Source: CAD feature listing. Evaluate the final solid. Frame: model axes, mm. A direction names the side the tool comes from. Coordinates: 2 decimals unless noted, no trailing zeros. Write each loop counter-clockwise with the first axis right and the second up, starting at its lowest first coordinate (ties: lowest second). Pieces come first, ordered by that corner, then holes. Notation, with made-up numbers: (-11, 76.25) -> (41, 76.25) arc R21 ccw to (41, 91.25) -> close; hole circle Ø4 at (53, -0.75). An arc over 180 degrees is marked (long way). One line per item, written item: value. Start each with the question number.
1. Mould query, pull axis X, two halves, no side actions, for faces 1 (the cylindrical face through (12.248, 5.151, -17.732)), 2 (the flat face through (0, 0, 2)), 3 (the flat face through (15, 0, -18)). Classes: released by +X, released by -X, zero draft, split by the parting line, or undercut.
2. Access query for faces 4 (the flat face through (5, 0, -7)), 5 (the cylindrical face through (-2.598, -3.237, 0.986)), 6 (the cylindrical face through (-4.4, 9.93, 1.01)), 7 (the flat face through (-2, 0, 0)), 8 (the flat face through (-8, 0, -18)). Directions: +Z, -Z, +X, -X, +Y, -Y. A direction counts if a zero-diameter tool reaches every point of the face in a straight line with its end or side. Return the directions, or none.
3. Section query C-C, the plane z = -4.5. Output: boundary loops of the cut face in (x, y).
4. Section query B-B, the plane y = -5.25. Output: boundary loops of the cut face in (x, z), and give its area (3 significant figures).
5. First-contact query: P1, Ø9, axis at y = 2, z = -10.5, coming from the +X side; P2, Ø1.9, axis at x = -2.26, y = 4.75, coming from the +Z side; P3, Ø8, axis at x = 12, z = -0.5, coming from the -Y side; P4, Ø1, axis at y = 1, z = 1.5, coming from the -X side. Flat tips, straight axial feed; report the tip coordinate or a pass-through.
6. Line query: line 1 (Y direction, x = 10, z = -17.75); line 2 (X direction, y = -5.25, z = -18.25); line 3 (Z direction, x = 0.75, y = 5.5). Output: solid intervals per line, ascending.
7. Section query A-A, the plane x = 10. Output: boundary loops of the cut face in (y, z), and give its area (3 significant figures).
Autodesk Fusion 360 part; units mm, degrees
sketch "Sketch1" plane through (0, 0, 0) normal (0, 0, 1) x (1, 0, 0)
  line L0 (5, 10.5) -> (-5, 10.5)
  line L1 (-5, 10.5) -> (-5, -10.5)
  line L2 (-5, -10.5) -> (5, -10.5)
  line L3 (5, -10.5) -> (5, 10.5)
  line L4 (5, 10.5) -> (-5, -10.5) construction
  line L5 (-5, 10.5) -> (5, -10.5) construction
  line L6 (5, -4.75) -> (-5, -4.75)
  line L7 (-5, -4.75) -> (-5, 4.75)
  line L8 (-5, 4.75) -> (5, 4.75)
  line L9 (5, 4.75) -> (5, -4.75)
  line L10 (5, -4.75) -> (-5, 4.75) construction
  line L11 (-5, -4.75) -> (5, 4.75) construction
  circle A0 centre (-2.2619, 4.75) radius 1.55
  circle A1 centre (-2.2619, -4.75) radius 1.55
  line L12 (5, 10.5) -> (2, 10.5)
  line L13 (2, 10.5) -> (2, -10.5)
  line L14 (2, -10.5) -> (5, -10.5)
  line L15 (5, -10.5) -> (5, 10.5)
  dimension "d1" = 10
  dimension "d2" = 21
  dimension "d3" = 10
  dimension "d4" = 9.5
  dimension "d5" = 3.1
  dimension "d6" = 3.1
  dimension "d7" = 3
extrude "Extrude1" add sketch "Sketch1" along normal blind 2 contours L0 L3 L8 L12 L13 L15 | L0 L1 L8 A0 L13 | L3 L6 L8 L9 L13 L15 | L1 L6 L7 L8 A0 A1 L13 | L2 L3 L6 L13 L14 L15 | L1 L2 L6 A1 L13
extrude "Extrude2" add sketch "Sketch1" against normal blind 19 contours L0 L3 L8 L12 L13 L15 | L3 L6 L8 L9 L13 L15 | L2 L3 L6 L13 L14 L15
sketch "Sketch2" plane through (5, 0, 0) normal (1, 0, 0) x (0, 1, 0)
  line L0 (10.5, -19) -> (10.5, 2)
  line L1 (10.5, 2) -> (-10.5, 2)
  line L2 (-10.5, 2) -> (-10.5, -19)
  line L3 (-10.5, -19) -> (10.5, -19)
  line L4 (-10.5, -19) -> (10.5, -19)
  line L5 (10.5, -19) -> (10.5, -16.5)
  line L6 (10.5, -16.5) -> (-10.5, -16.5)
  line L7 (-10.5, -16.5) -> (-10.5, -19)
  dimension "d12" = 2.5
extrude "Extrude3" add sketch "Sketch2" along normal blind 10 and the other way blind 13 contours L0 L2 L3 L4 L5 L6 L7
sketch "Sketch3" plane through (0, 0, -16.5) normal (0, 0, 1) x (-1, 0, 0)
  line L0 (-5, -10.5) -> (-5, 10.5)
  line L1 (-5, 10.5) -> (-15, 10.5)
  line L2 (-15, 10.5) -> (-15, -10.5)
  line L3 (-15, -10.5) -> (-5, -10.5)
  line L4 (-10, -10.5) -> (-10, 10.5)
  line L5 (-15, 0) -> (-5, 0)
  line L6 (-10, 0) -> (-10, -10.5)
  circle A0 centre (-10, -5.25) radius 2.25
  line L7 (-10, 0) -> (-10, 10.5)
  circle A1 centre (-10, 5.25) radius 2.25
  dimension "d17" = 4.5
  dimension "d18" = 4.5
fillet "Fillet1" radius 2 6 edges at (15, -10.5, -17.75) (15, 10.5, -17.75) (-8, -10.5, -17.75) (-5, -10.5, 1) (-5, 10.5, 1) (-8, 10.5, -17.75)
extrude "Extrude4" cut sketch "Sketch3" against normal blind 7 contours L4 L6 A0 | L4 L6 A0 | L4 L7 A1 | L4 L7 A1
Computed values:
1. face 1: undercut
1. face 2: zero draft
1. face 3: released by +X
2. face 4: +Z, +X, +Y, -Y
2. face 5: +Z
2. face 6: +Z, -X, +Y
2. face 7: -X, +Y, -Y
2. face 8: +Z, -Z, -X, +Y, -Y
3. outline: (2, -10.5) -> (5, -10.5) -> (5, 10.5) -> (2, 10.5) -> close
4. outline: (-8, -19) -> (7.75, -19) -> (7.75, -16.5) -> (5, -16.5) -> (5, 2) -> (-0.79, 2) -> (-0.79, 0) -> (2, 0) -> (2, -16.5) -> (-8, -16.5) -> close; (-5, 0) -> (-3.73, 0) -> (-3.73, 2) -> (-5, 2) -> close; (12.25, -19) -> (15, -19) -> (15, -16.5) -> (12.25, -16.5) -> close
4. area: 110 mm²
5. P1: stops at x = 5
5. P2: stops at z = -16.5
5. P3: passes through
5. P4: stops at x = -5
6. line 1: y = -10.5 to -7.5, -3 to 3, 7.5 to 10.5
6. line 2: x = -8 to 7.75, 12.25 to 15
6. line 3: z = -19 to -16.5, 0 to 2
7. outline: (-10.5, -19) -> (-7.5, -19) -> (-7.5, -16.5) -> (-10.5, -16.5) -> close; (-3, -19) -> (3, -19) -> (3, -16.5) -> (-3, -16.5) -> close; (7.5, -19) -> (10.5, -19) -> (10.5, -16.5) -> (7.5, -16.5) -> close
7. area: 30.0 mm²
